Could you check a few things on this model? Use its own coordinates, in mm. Round coordinates to 2 decimals unless told otherwise and drop trailing zeros. Order: outer loops, then holes, each group sorted by start corner. A loop starts at its lowest first (then second) coordinate and runs counter-clockwise, first axis right, second up. Notation, with made-up numbers: (60, -26.5) - (115, -26.5) arc R13 ccw to (115, -19.5) - close; hole circle Ø9 at (88.5, 12.25). An arc over 180 degrees is marked (long way). Use one line per item in the form item = value.
from build123d import *

# Parameters (mm, degrees)
SKETCH1_R           = 2.4257
BOSS_EXTRUDE1_DEPTH = 3.175


with BuildPart() as part:
    # Sketch1 → Boss-Extrude1 (new body)
    with BuildSketch(Plane(origin=(0, 0, 0), x_dir=(1, 0, 0), z_dir=(0, 1, 0))):
        Polygon((0, 0), (0, 139.7), (38.1, 139.7), (161.789864335, 38.1), (161.789864335, 0), align=None)
        with Locations(Location((31.75, 15.875, 0), (0, 0, 270))):
            Circle(SKETCH1_R, mode=Mode.SUBTRACT)
        with Locations(Location((82.55, 15.875, 0), (0, 0, 270))):
            Circle(SKETCH1_R, mode=Mode.SUBTRACT)
        with Locations(Location((133.35, 15.875, 0), (0, 0, 270))):
            Circle(SKETCH1_R, mode=Mode.SUBTRACT)
        with Locations(Location((16.891, 53.975, 0), (0, 0, 270))):
            Circle(SKETCH1_R, mode=Mode.SUBTRACT)
        with Locations(Location((16.891, 79.375, 0), (0, 0, 270))):
            Circle(SKETCH1_R, mode=Mode.SUBTRACT)
        with Locations(Location((16.891, 104.775, 0), (0, 0, 270))):
            Circle(SKETCH1_R, mode=Mode.SUBTRACT)
        with Locations(Location((16.891, 130.175, 0), (0, 0, 270))):
            Circle(SKETCH1_R, mode=Mode.SUBTRACT)
    extrude(amount=BOSS_EXTRUDE1_DEPTH)


solid = part.part
Item 1: Imagine slicing it at D-D on z = -16. Please give me the cut outline in (x, y) (3 decimals), plus the area to 3 significant figures.
Found:
outline = (0, 0) - (29.328, 0) - (29.328, 3.175) - (0, 3.175) - close; (34.172, 0) - (80.128, 0) - (80.128, 3.175) - (34.172, 3.175) - close; (84.972, 0) - (130.928, 0) - (130.928, 3.175) - (84.972, 3.175) - close; (135.772, 0) - (161.79, 0) - (161.79, 3.175) - (135.772, 3.175) - close
area = 468 mm2
Item 2: If we mould it in two halves opening along X, with no side actions, what happens to faces 1 (the face through (99.08, 1.57, -89.61)), 2 (the face through (64, 0, -55)), 3 (the face through (17.62, 1.57, -127.86))? For each: released by +X, released by -X, zero draft, split by the parting line, or undercut.
Found:
face_1 = released by +X
face_2 = zero draft
face_3 = undercut
Item 3: Imagine slicing it at B-B on z = -105. Please give me the cut outline in (x, y) (3 decimals).
Found:
outline = (0, 0) - (14.476, 0) - (14.476, 3.175) - (0, 3.175) - close; (19.306, 0) - (80.344, 0) - (80.344, 3.175) - (19.306, 3.175) - close
Item 4: Imagine slicing it at A-A on x = 31.75. Please give me the cut outline in (y, z) (3 decimals), plus the area to 3 significant figures.
Found:
outline = (0, -139.7) - (3.175, -139.7) - (3.175, -18.301) - (0, -18.301) - close; (0, -13.449) - (3.175, -13.449) - (3.175, 0) - (0, 0) - close
area = 428 mm2
Item 5: Imagine slicing it at C-C on y = 2.25. Please give me the cut outline in (x, z) (3 decimals).
Found:
outline = (0, -139.7) - (38.1, -139.7) - (161.79, -38.1) - (161.79, 0) - (0, 0) - close; hole circle Ø4.851 at (16.891, -130.175); hole circle Ø4.851 at (16.891, -104.775); hole circle Ø4.851 at (16.891, -79.375); hole circle Ø4.851 at (16.891, -53.975); hole circle Ø4.851 at (31.75, -15.875); hole circle Ø4.851 at (82.55, -15.875); hole circle Ø4.851 at (133.35, -15.875)
Item 6: I need wall thicknesses on L1, parallel to X at y = 0.95, z = -57; L2, parallel to Z at x = 66.5, y = 2.3; L3, parallel to X at y = 1.05, z = -66. Which ranges of each line are inside material? Lowest first, please.
Found:
L1 = 0 to 138.78
L2 = -116.37 to 0
L3 = 0 to 127.82
Item 7: Will these pins go through, and if not, where does the flat tip stop? P1, Ø4, axis at x = 16.891, z = -53.975, coming from the +Y side; P2, Ø1, axis at y = 2, z = -108.5, coming from the +X side; P3, Ø10, axis at x = 105.5, z = -59, coming from the -Y side.
Found:
P1 = through
P2 = 76.69
P3 = 0
